Autodesk Inventor part; units mm, degrees
ref_plane "YZ Plane" through (0, 0, 0) normal (1, 0, 0) x (0, 1, 0)
ref_plane "XZ Plane" through (0, 0, 0) normal (0, 1, 0) x (-1, 0, 0)
ref_plane "XY Plane" through (0, 0, 0) normal (0, 0, 1) x (1, 0, 0)
sketch "スケッチ1" plane through (0, 0, 0) normal (0, 0, 1) x (1, 0, 0)
  line L0 (-70, 75) -> (70, 75)
  line L1 (70, 75) -> (70, -75)
  line L2 (70, -75) -> (-70, -75)
  line L3 (-70, -75) -> (-70, 75)
  line L4 (70, 92.6777) -> (87.6777, 75)
  line L5 (87.6777, 75) -> (70, 57.3223)
  line L6 (70, 57.3223) -> (52.3223, 75)
  line L7 (52.3223, 75) -> (70, 92.6777)
  line L8 (70, -57.3223) -> (87.6777, -75)
  line L9 (87.6777, -75) -> (70, -92.6777)
  line L10 (70, -92.6777) -> (52.3223, -75)
  line L11 (52.3223, -75) -> (70, -57.3223)
  line L12 (-70, -57.3223) -> (-52.3223, -75)
  line L13 (-52.3223, -75) -> (-70, -92.6777)
  line L14 (-70, -92.6777) -> (-87.6777, -75)
  line L15 (-87.6777, -75) -> (-70, -57.3223)
  line L16 (-70, 92.6777) -> (-52.3223, 75)
  line L17 (-52.3223, 75) -> (-70, 57.3223)
  line L18 (-70, 57.3223) -> (-87.6777, 75)
  line L19 (-87.6777, 75) -> (-70, 92.6777)
  point P0 (0, 0)
  point P1 (70, 75)
  dimension "d0" = 150
  dimension "d1" = 75
  dimension "d2" = 140
  dimension "d3" = 70
  dimension "d4" = 12.5
  dimension "d5" = 12.5
  dimension "d6" = 12.5
  dimension "d7" = 12.5
extrude "押し出し1" add sketch "スケッチ1" along normal blind 3
sketch "スケッチ2" plane through (0, 0, 3) normal (0, 0, 1) x (1, 0, 0)
  line L0 (87.6777, 75) -> (70, 57.3223)
  line L1 (70, 92.6777) -> (87.6777, 75)
  line L2 (52.3223, 75) -> (70, 92.6777)
  line L3 (-70, 92.6777) -> (-52.3223, 75)
  line L4 (-87.6777, 75) -> (-70, 92.6777)
  line L5 (-70, 57.3223) -> (-87.6777, 75)
  line L6 (-87.6777, -75) -> (-70, -57.3223)
  line L7 (-70, -92.6777) -> (-87.6777, -75)
  line L8 (-52.3223, -75) -> (-70, -92.6777)
  line L9 (70, -92.6777) -> (52.3223, -75)
  line L10 (87.6777, -75) -> (70, -92.6777)
  line L11 (70, -57.3223) -> (87.6777, -75)
  circle A0 centre (-56.2114, -49.8977) radius 1.5
  circle A1 centre (-44.8977, -61.2114) radius 1.5
  circle A2 centre (44.8977, -61.2114) radius 1.5
  circle A3 centre (56.2114, -49.8977) radius 1.5
  circle A4 centre (56.2114, 49.8977) radius 1.5
  circle A5 centre (44.8977, 61.2114) radius 1.5
  circle A6 centre (-44.8977, 61.2114) radius 1.5
  circle A7 centre (-56.2114, 49.8977) radius 1.5
  point P0 (0, 0)
  dimension "d10" = 3
  dimension "d12" = 40
  dimension "d13" = 40
  dimension "d14" = 4.5
  dimension "d15" = 4.5
  dimension "d16" = 40
  dimension "d17" = 40
  dimension "d18" = 40
  dimension "d19" = 40
  dimension "d20" = 40
  dimension "d21" = 40
  dimension "d22" = 4.5
  dimension "d23" = 4.5
  dimension "d24" = 4.5
  dimension "d25" = 4.5
  dimension "d26" = 4.5
  dimension "d27" = 4.5
hole "穴1" at (44.8977, -61.2114, 3) at (56.2114, -49.8977, 3) at (-44.8977, -61.2114, 3) at (-56.2114, -49.8977, 3) at (44.8977, 61.2114, 3) at (56.2114, 49.8977, 3) at (-56.2114, 49.8977, 3) at (-44.8977, 61.2114, 3) direction (0, 0, -1) diameter 3 end through all
sketch "スケッチ3" plane through (0, 0, 3) normal (0, 0, 1) x (1, 0, 0)
  line L0 (87.6777, 75) -> (70, 57.3223)
  line L1 (70, 92.6777) -> (87.6777, 75)
  line L2 (52.3223, 75) -> (70, 92.6777)
  line L3 (-70, 92.6777) -> (-52.3223, 75)
  line L4 (-87.6777, 75) -> (-70, 92.6777)
  line L5 (-70, 57.3223) -> (-87.6777, 75)
  line L6 (-87.6777, -75) -> (-70, -57.3223)
  line L7 (-70, -92.6777) -> (-87.6777, -75)
  line L8 (-52.3223, -75) -> (-70, -92.6777)
  line L9 (70, -92.6777) -> (52.3223, -75)
  line L10 (87.6777, -75) -> (70, -92.6777)
  line L11 (70, -57.3223) -> (87.6777, -75)
  circle A0 centre (-49.1403, 65.4541) radius 2.25
  circle A1 centre (-60.4541, 54.1403) radius 2.25
  circle A2 centre (-60.4541, -54.1403) radius 2.25
  circle A3 centre (-49.1403, -65.4541) radius 2.25
  circle A4 centre (49.1403, -65.4541) radius 2.25
  circle A5 centre (60.4541, -54.1403) radius 2.25
  circle A6 centre (60.4541, 54.1403) radius 2.25
  circle A7 centre (49.1403, 65.4541) radius 2.25
  point P0 (0, 0)
  dimension "d35" = 4.5
  dimension "d37" = 4.5
  dimension "d38" = 4.5
  dimension "d39" = 34
  dimension "d40" = 34
  dimension "d41" = 4.5
  dimension "d42" = 4.5
  dimension "d43" = 34
  dimension "d44" = 34
  dimension "d45" = 34
  dimension "d46" = 4.5
  dimension "d47" = 4.5
  dimension "d48" = 34
  dimension "d49" = 34
  dimension "d50" = 34
  dimension "d51" = 4.5
  dimension "d52" = 4.5
hole "穴2" at (-60.4541, -54.1403, 3) at (-49.1403, -65.4541, 3) at (49.1403, 65.4541, 3) at (60.4541, 54.1403, 3) at (-60.4541, 54.1403, 3) at (-49.1403, 65.4541, 3) at (49.1403, -65.4541, 3) at (60.4541, -54.1403, 3) direction (0, 0, -1) diameter 4.5 end through all
sketch "スケッチ4" plane through (0, 0, 3) normal (0, 0, 1) x (1, 0, 0)
  line L0 (87.6777, 75) -> (70, 57.3223)
  line L1 (70, 92.6777) -> (87.6777, 75)
  line L2 (52.3223, 75) -> (70, 92.6777)
  line L3 (-70, 92.6777) -> (-52.3223, 75)
  line L4 (-87.6777, 75) -> (-70, 92.6777)
  line L5 (-70, 57.3223) -> (-87.6777, 75)
  line L6 (-87.6777, -75) -> (-70, -57.3223)
  line L7 (-70, -92.6777) -> (-87.6777, -75)
  line L8 (-52.3223, -75) -> (-70, -92.6777)
  line L9 (70, -92.6777) -> (52.3223, -75)
  line L10 (87.6777, -75) -> (70, -92.6777)
  line L11 (70, -57.3223) -> (87.6777, -75)
  line L12 (-70, -57.3223) -> (-52.3223, -75)
  line L13 (52.3223, -75) -> (70, -57.3223)
  line L14 (52.3223, 75) -> (70, 57.3223)
  line L15 (-70, 57.3223) -> (-52.3223, 75)
  point P0 (0, 0)
  dimension "d60" = 25
  dimension "d61" = 25
  dimension "d62" = 25
  dimension "d63" = 25
extrude "押し出し2" cut sketch "スケッチ4" against normal blind 3
sketch "スケッチ6" plane through (-52.3223, 75, 0) normal (0, 1, 0) x (1, 0, 0)
  line L0 (104.6447, 0) -> (0, 0)
  line L1 (0, -3) -> (104.6447, -3)
  line L2 (39.8223, 0) -> (64.8223, 0)
  line L3 (64.8223, 0) -> (64.8223, -3)
  line L4 (64.8223, -3) -> (39.8223, -3)
  line L5 (39.8223, -3) -> (39.8223, 0)
  point P0 (52.3223, 0)
  dimension "d66" = 25
  dimension "d68" = 12.5
extrude "押し出し3" add sketch "スケッチ6" along normal blind 10
sketch "スケッチ7" plane through (0, 0, 3) normal (0, 0, 1) x (1, 0, 0)
  line L0 (-12.5, 85) -> (12.5, 85)
  line L1 (-12.5, 75) -> (-12.5, 85)
  circle A0 centre (-8, 73) radius 1.5
  circle A1 centre (8, 73) radius 1.5
  point P0 (0, 0)
  dimension "d71" = 16
  dimension "d72" = 12
  dimension "d73" = 12
  dimension "d74" = 3
  dimension "d75" = 4.5
hole "穴3" at (-8, 73, 3) at (8, 73, 3) direction (0, 0, -1) diameter 3 end through all
sketch "スケッチ9" plane through (0, 0, 3) normal (0, 0, 1) x (1, 0, 0)
  line L0 (52.3223, -75) -> (-52.3223, -75)
  circle A0 centre (-32.5, -61.5) radius 1.5
  circle A1 centre (-32.5, -28.5) radius 1.5
  circle A2 centre (-32.5, 4.5) radius 1.5
  circle A3 centre (32.5, -61.5) radius 1.5
  circle A4 centre (32.5, -28.5) radius 1.5
  circle A5 centre (32.5, 4.5) radius 1.5
  point P0 (0, 0)
  dimension "d95" = 3
  dimension "d97" = 13.5
  dimension "d98" = 33
  dimension "d99" = 33
  dimension "d100" = 33
  dimension "d101" = 33
  dimension "d102" = 13.5
  dimension "d103" = 65
  dimension "d104" = 65
  dimension "d105" = 65
  dimension "d106" = 32.5
  dimension "d107" = 32.5
  dimension "d108" = 32.5
hole "穴5" at (-32.5, 4.5, 3) at (-32.5, -28.5, 3) at (-32.5, -61.5, 3) at (32.5, -61.5, 3) at (32.5, -28.5, 3) at (32.5, 4.5, 3) direction (0, 0, -1) diameter 3 end through all
sketch "スケッチ10" plane through (0, 0, 3) normal (0, 0, 1) x (1, 0, 0)
  circle A0 centre (-20, 57) radius 1.5
  circle A1 centre (20, 57) radius 1.5
  circle A2 centre (-20, 25) radius 1.5
  circle A3 centre (20, 25) radius 1.5
  point P0 (0, 0)
  dimension "d116" = 3
  dimension "d118" = 40
  dimension "d119" = 32
  dimension "d120" = 40
  dimension "d122" = 20
  dimension "d123" = 25
  dimension "d124" = 25
  dimension "d125" = 32
  dimension "d126" = 20
hole "穴6" at (-20, 57, 3) at (-20, 25, 3) at (20, 25, 3) at (20, 57, 3) direction (0, 0, -1) diameter 3 end through all
equation "\"d33\" = d26"
equation "\"d58\" = d46"
properties material "アルミニウム 6061"
Check sheet for the modelled part. Datum: model origin and axes. Units: mm. Give positions to 0.01 mm unless a question says otherwise; leave off trailing zeros. Write each loop counter-clockwise with the first axis right and the second up, starting at its lowest first coordinate (ties: lowest second). Pieces come first, ordered by that corner, then holes. Notation, with made-up numbers: (47, 19) - (105, 19) arc R35 cw to (105, 53) - close; hole circle Ø7 at (-18, 47.25). An arc over 180 degrees is marked (long way). Answer as a JSON object with one key per item and string values. Group by question number.
1) Sectioned sample at A-A (x = -39). Record the cut outline in (y, z), then the cut area to 3 significant figures.
2) Depth check by flat-ended pin: P1, Ø1.5, axis at x = 15.5, z = 2, coming from the +Y side. Enter the tip coordinate at first touch or a pass-through.
3) Release check for a two-part mould opening along X. For faces 1 (the face through (-61.28, 66.04, 1.52)), 2 (the face through (-51.37, 65.75, 1.48)), 3 (the face through (-1, 6, 3)) record: pulls with the +X half, pulls with the -X half, needs draft (parallel to the pull), parting line crosses it, or undercut.
4) Thickness scan on probe 1 along Y at (x, z) = (-32.5, 0.75); probe 2 along X at (y, z) = (-28.5, 2.2); probe 3 along X at (y, z) = (57, 0.8). Record the ranges inside material, lowest first. Write a range as from..to.
5) Sectioned sample at B-B (z = 1.7). Give the number of separate pieces and of enclosed holes in the cut face, then the cut area to 3 significant figures.
Geometry results:
{
 "1": {"outline": "(-75, 0) - (75, 0) - (75, 3) - (-75, 3) - close", "area": "450 mm^2"},
 "2": {"P1": "stops at y = 75"},
 "3": {"face 1": "pulls with the -X half", "face 2": "undercut", "face 3": "needs draft"},
 "4": {"probe 1": "y = -75..-63, -60..-30, -27..3, 6..75", "probe 2": "x = -70..-34, -31..31, 34..70", "probe 3": "x = -70..-21.5, -18.5..18.5, 21.5..70"},
 "5": {"separate pieces": "1", "enclosed holes": "28", "area": "20,400 mm^2"}
}
